Input: dimensioned drawing with shaded views. Units: mm. Origin: part minimum x, y, z. A direction names the side the tool comes from. Round coordinates to 2 decimals unless told otherwise and drop trailing zeros. Write each loop counter-clockwise with the first axis right and the second up, starting at its lowest first coordinate (ties: lowest second). Pieces come first, ordered by that corner, then holes. Notation, with made-up numbers: (50, -11.5) -> (86, -11.5) arc R26 cw to (86, 13.5) -> close; hole circle Ø6 at (53.5, 0.5). An arc over 180 degrees is marked (long way). Return JSON: item names as keys, results as strings. Group by question number.
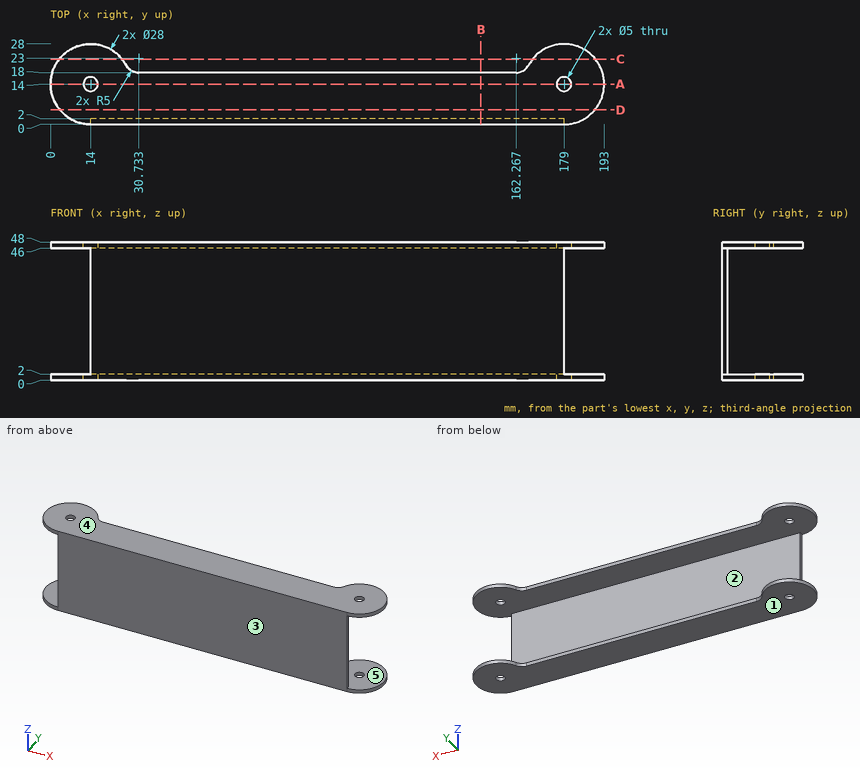
Item 1: Cut plane C-C on y = 22.75. Output: boundary loops of the cut face in (x, z), and give its area (3 significant figures).
Item 2: First-contact query: pin 1 Ø10 at (y, z) = (23, 42) entering from -X; pin 2 Ø1.6 at (y, z) = (1, 19.5) entering from -X; pin 3 Ø6 at (x, y) = (14, 14) entering from -Z; pin 4 Ø22 at (x, z) = (88.5, 16.5) entering from +Y. Flat tips, straight axial feed; report the tip coordinate or a pass-through.
Item 3: Material intervals for probe 1 along Z at (x, y) = (40.5, 14); probe 2 along Y at (x, z) = (179, 0.8); probe 3 along Y at (x, z) = (45.5, 22), sorted ascending.
Item 4: Pull-direction query (Z, two-part tool) for the marked faces 3, 4 and 5; classes: +Z half, -Z half, draft (parallel to the pull), parting line (faces both ways), or undercut.
Item 5: Cut plane A-A on y = 14. Output: boundary loops of the cut face in (x, z), and give its area (3 significant figures).
Item 6: Cut plane D-D on y = 5. Output: boundary loops of the cut face in (x, z).
Item 7: Cut plane B-B on x = 150. Output: boundary loops of the cut face in (y, z), and give its area (3 significant figures).
Item 8: Set-up query: the marked faces 1 and 2. Return all of +Z, -Z, +X, -X, +Y, -Y with unobstructed straight access to the full face (end or side cutting, diameter ignored); none if empty.
Here are the results:
{
 "1": {"outline": "(3.07, 0) -> (24.93, 0) -> (24.93, 2) -> (3.07, 2) -> close; (3.07, 46) -> (24.93, 46) -> (24.93, 48) -> (3.07, 48) -> close; (168.07, 0) -> (189.93, 0) -> (189.93, 2) -> (168.07, 2) -> close; (168.07, 46) -> (189.93, 46) -> (189.93, 48) -> (168.07, 48) -> close", "area": "175 mm^2"},
 "2": {"pin 1": "stops at x = 1.35", "pin 2": "stops at x = 14", "pin 3": "stops at z = 0", "pin 4": "stops at y = 2"},
 "3": {"probe 1": "z = 0 to 2, 46 to 48", "probe 2": "y = 0 to 11.5, 16.5 to 28", "probe 3": "y = 0 to 2"},
 "4": {"face 3": "draft", "face 4": "+Z half", "face 5": "undercut"},
 "5": {"outline": "(0, 0) -> (11.5, 0) -> (11.5, 2) -> (0, 2) -> close; (0, 46) -> (11.5, 46) -> (11.5, 48) -> (0, 48) -> close; (16.5, 0) -> (176.5, 0) -> (176.5, 2) -> (16.5, 2) -> close; (16.5, 46) -> (176.5, 46) -> (176.5, 48) -> (16.5, 48) -> close; (181.5, 0) -> (193, 0) -> (193, 2) -> (181.5, 2) -> close; (181.5, 46) -> (193, 46) -> (193, 48) -> (181.5, 48) -> close", "area": "732 mm^2"},
 "6": {"outline": "(3.28, 0) -> (189.72, 0) -> (189.72, 2) -> (3.28, 2) -> close; (3.28, 46) -> (189.72, 46) -> (189.72, 48) -> (3.28, 48) -> close"},
 "7": {"outline": "(0, 0) -> (18, 0) -> (18, 2) -> (2, 2) -> (2, 46) -> (18, 46) -> (18, 48) -> (0, 48) -> close", "area": "160 mm^2"},
 "8": {"face 1": "-Z, +X, -X, +Y, -Y", "face 2": "+X, -X, +Y"}
}
